```python
from build123d import *

# Parameters (mm, degrees)
F0_W     = 0.762
F0_H     = 1.27
F1_DEPTH = 12.7
F2_R     = 2.54
F3_DEPTH = 4.446


with BuildPart() as f1:
    # F0 (on Front) → F1 (new body, symmetric)
    with BuildSketch(Plane.XZ):
        Polygon((11.938, 1.5875), (-12.7, 1.5875), (-12.7, -1.5875), (12.7, -1.5875), (12.7, 1.5875), align=None)
        with Locations((12.319, 2.2225)):
            Rectangle(F0_W, F0_H)
    extrude(amount=F1_DEPTH, both=True)

    # F2 (on face) → F3 (cut, through all)
    with BuildSketch(Plane(origin=(0, 0, -1.5875), x_dir=(1, 0, 0), z_dir=(0, 0, -1))):
        with Locations((-7.62, 7.62)):
            Circle(F2_R)
        with Locations((-7.62, -7.62)):
            Circle(F2_R)
    extrude(amount=-F3_DEPTH, mode=Mode.SUBTRACT)


solid = f1.part
```
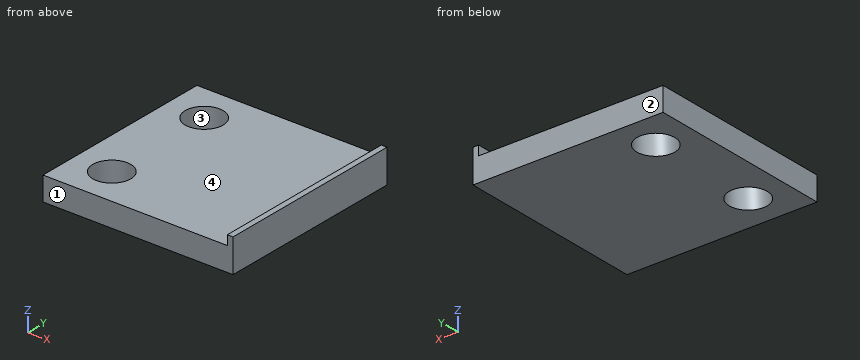
Can you work these out from the model? Positions are in its coordinate system, mm. Face numbers are marked on the shaded views. Give positions to 0.01 mm unless a question says otherwise; leave off trailing zeros. Loops run counter-clockwise (first coordinate to the right, second up) from the corner with the lowest first, then second, coordinate; pieces in that order, holes last. Notation, with made-up numbers: M -0.75,20 L 30.25,20 A25 cw 30.25,48 Z; hole C 7,-39.75 d2. An arc over 180 degrees is marked long. One line per item, written item: value.
(1) Suppose I cut it at D-D on y = 3. List the corners of the cut face in (x, z) for me, plus the area to 3 significant figures.
Returned:
outline: M -12.7,-1.59 L 12.7,-1.59 L 12.7,2.86 L 11.94,2.86 L 11.94,1.59 L -12.7,1.59 Z
area: 81.6 mm^2
(2) We'd pull the mould along Y, two halves only. Please class the marked faces 1, 2, 3 and 4: released by +Y, released by -Y, zero draft, split by the parting line, or undercut.
Returned:
face 1: released by -Y
face 2: released by +Y
face 3: undercut
face 4: zero draft
(3) Suppose I cut it at B-B on x = -7.62. List the corners of the cut face in (y, z) for me.
Returned:
outline: M -12.7,-1.59 L -10.16,-1.59 L -10.16,1.59 L -12.7,1.59 Z; M -5.08,-1.59 L 5.08,-1.59 L 5.08,1.59 L -5.08,1.59 Z; M 10.16,-1.59 L 12.7,-1.59 L 12.7,1.59 L 10.16,1.59 Z
(4) Suppose I cut it at A-A on y = -7.62. List the corners of the cut face in (x, z) for me, plus the area to 3 significant figures.
Returned:
outline: M -12.7,-1.59 L -10.16,-1.59 L -10.16,1.59 L -12.7,1.59 Z; M -5.08,-1.59 L 12.7,-1.59 L 12.7,2.86 L 11.94,2.86 L 11.94,1.59 L -5.08,1.59 Z
area: 65.5 mm^2
(5) Will these pins go through, and if not, where does the flat tip stop? pin 1 (8 mm diameter, centred on x = -7.62, y = 7.62, fed in from -Z); pin 2 (2 mm diameter, centred on x = -5, y = -6.5, fed in from +Z); pin 3 (3 mm diameter, centred on x = -7.62, y = -7.62, fed in from -Z).
Returned:
pin 1: z = -1.59
pin 2: z = 1.59
pin 3: through
(6) I need wall thicknesses on line 1 (Y direction, x = -7.62, z = 0.9); line 2 (X direction, y = -7.62, z = 0.6); line 3 (Y direction, x = -8, z = 1.1). Which ranges of each line are inside material? Lowest first, please.
Returned:
line 1: -12.7 to -10.16, -5.08 to 5.08, 10.16 to 12.7
line 2: -12.7 to -10.16, -5.08 to 12.7
line 3: -12.7 to -10.13, -5.11 to 5.11, 10.13 to 12.7
(7) Suppose I cut it at C-C on z = 0. List the corners of the cut face in (x, y) for me.
Returned:
outline: M -12.7,-12.7 L 12.7,-12.7 L 12.7,12.7 L -12.7,12.7 Z; hole C -7.62,-7.62 d5.08; hole C -7.62,7.62 d5.08
